```python
from build123d import *

# Parameters (mm, degrees)
ESBO_O1_R                = 10
RESSALTO_EXTRUS_O1_DEPTH = 7.6
FURO1_D                  = 26.4
FURO1_DEPTH              = 2.4
ESBO_O7_OUTSIDE_W        = 110.904
ESBO_O7_OUTSIDE_H        = 115.328
ESBO_O7_OUTSIDE_R        = 14.3
CORTE_EXTRUS_O1_DEPTH    = 13
CORTE_EXTRUS_O1_DRAFT    = -70
ESBO_O8_OUTSIDE_W        = 110.904
ESBO_O8_OUTSIDE_H        = 115.328
ESBO_O8_OUTSIDE_R        = 14.3
CORTE_EXTRUS_O2_DEPTH    = 13
CORTE_EXTRUS_O2_DRAFT    = -70


with BuildPart() as part:
    # Esboço1 → Ressalto-extrusão1 (new body)
    with BuildSketch(Plane(origin=(0, 0, 0), x_dir=(0, 0, -1), z_dir=(1, 0, 0))):
        Polygon((14.3, 8.256108849), (0, 16.512217699), (-14.3, 8.256108849), (-14.3, -8.256108849), (0, -16.512217699), (14.3, -8.256108849), align=None)
        with Locations(Location((0, 0, 0), (0, 0, 180))):
            Circle(ESBO_O1_R, mode=Mode.SUBTRACT)
    extrude(amount=RESSALTO_EXTRUS_O1_DEPTH)

    # Furo1
    with Locations(Plane(origin=(7.6, 0, 0), x_dir=(0, 0, -1), z_dir=(1, 0, 0))):
        with Locations((0, 0)):
            Hole(FURO1_D / 2, depth=FURO1_DEPTH)


with BuildPart() as corte_extrus_o1_tool:
    # Esboço7 outside → Corte-extrusão1 (with draft: the straight prism first)
    with BuildSketch(Plane(origin=(7.6, 0, 0), x_dir=(0, 0, -1), z_dir=(1, 0, 0))):
        Rectangle(ESBO_O7_OUTSIDE_W, ESBO_O7_OUTSIDE_H)
        Circle(ESBO_O7_OUTSIDE_R, mode=Mode.SUBTRACT)
    extrude(amount=-CORTE_EXTRUS_O1_DEPTH)
    # Corte-extrusão1: the draft: its side faces are tilted about the plane it starts from
    corte_extrus_o1_sides = [corte_extrus_o1_tool.faces().sort_by_distance(p)[0] for p in [
        (1.1, -57.664, 0),
        (1.1, 0, -55.452),
        (1.1, 57.664, 0),
        (1.1, 0, 55.452),
        (1.1, 0, 14.3),
    ]]
    draft(corte_extrus_o1_sides, Plane(origin=(7.6, 0, 0), x_dir=(0, 0, -1), z_dir=(1, 0, 0)), CORTE_EXTRUS_O1_DRAFT)


with BuildPart() as part_1:
    add(part.part)

    # Corte-extrusão1: cut by corte_extrus_o1_tool
    add(corte_extrus_o1_tool.part, mode=Mode.SUBTRACT)


with BuildPart() as corte_extrus_o2_tool:
    # Esboço8 outside → Corte-extrusão2 (with draft: the straight prism first)
    with BuildSketch(Plane.ZY):
        Rectangle(ESBO_O8_OUTSIDE_W, ESBO_O8_OUTSIDE_H)
        Circle(ESBO_O8_OUTSIDE_R, mode=Mode.SUBTRACT)
    extrude(amount=-CORTE_EXTRUS_O2_DEPTH)
    # Corte-extrusão2: the draft: its side faces are tilted about the plane it starts from
    corte_extrus_o2_sides = [corte_extrus_o2_tool.faces().sort_by_distance(p)[0] for p in [
        (6.5, -57.664, 0),
        (6.5, 0, 55.452),
        (6.5, 57.664, 0),
        (6.5, 0, -55.452),
        (6.5, 0, -14.3),
    ]]
    draft(corte_extrus_o2_sides, Plane.ZY, CORTE_EXTRUS_O2_DRAFT)


with BuildPart() as part_2:
    add(part_1.part)

    # Corte-extrusão2: cut by corte_extrus_o2_tool
    add(corte_extrus_o2_tool.part, mode=Mode.SUBTRACT)


solid = part_2.part
```
Source: CAD feature listing. Evaluate the final solid. Frame: model axes, mm. Coordinates: 2 decimals unless noted, no trailing zeros. Order: outer loops, then holes, each group sorted by start corner. A loop starts at its lowest first (then second) coordinate and runs counter-clockwise, first axis right, second up. Notation, with made-up numbers: (-31.75, 87) - (8.25, 87) arc R25 cw to (8.25, 114) - close; hole circle Ø7 at (-27.5, -25). An arc over 180 degrees is marked (long way). One line per item, written item: value.
1) Mould query, pull axis Y, two halves, no side actions, for faces 1 (the face through (3.747, -12.326, 7.25)), 2 (the face through (4, 0, -14.3)), 3 (the face through (6.38, 8.92, -9.73)). Classes: released by +Y, released by -Y, zero draft, split by the parting line, or undercut.
Computed values:
face 1: released by -Y
face 2: zero draft
face 3: undercut
2) Contact query for a flat-ended pin moving along its axis: pin 1 (5 mm diameter, centred on y = 2, z = 8, fed in from +X). Output: stop coordinate, or through.
Computed values:
pin 1: stops at x = 5.2
3) Ray query, line 1 (Y direction, x = 3.65, z = 0); line 2 (Y direction, x = 6.7, z = 0); line 3 (X direction, y = -8, z = -10). Return the intervals inside material, ascending. Write a range as [from, to].
Computed values:
line 1: y = [-16.51, -10], [10, 16.51]
line 2: y = [-16.51, -13.2], [13.2, 16.51]
line 3: x = [0, 5.2]
4) Cut plane A-A on x = 1.5. Output: boundary loops of the cut face in (y, z).
Computed values:
outline: (-16.51, 0) - (-8.26, -14.3) - (8.26, -14.3) - (16.51, 0) - (8.26, 14.3) - (-8.26, 14.3) - close; hole circle Ø20 at (0, 0)
